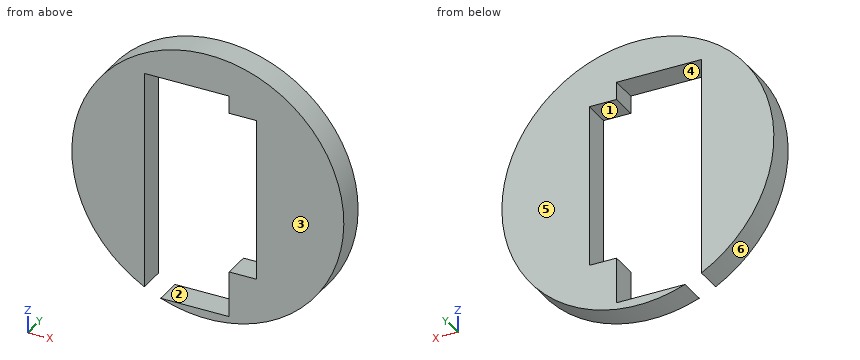
```python
from build123d import *

# Parameters (mm, degrees)
SKETCH1_R           = 47.625
BOSS_EXTRUDE1_DEPTH = 12.7
SKETCH2_R           = 47.625
BOSS_EXTRUDE4_DEPTH = 12.7
BOSS_EXTRUDE5_DEPTH = 4.7625
SKETCH14_W          = 19.812
SKETCH14_H          = 52.959
CUT_EXTRUDE11_DEPTH = 9.275815586
BOSS_EXTRUDE7_DEPTH = 6.35


with BuildPart() as part:
    # Sketch1 → Boss-Extrude1 (new body)
    with BuildSketch(Plane(origin=(0, 0, 0), x_dir=(1, 0, 0), z_dir=(0, 1, 0))):
        Circle(SKETCH1_R)
    extrude(amount=-BOSS_EXTRUDE1_DEPTH)

    # Sketch14 → Cut-Extrude11 (cut)
    with BuildSketch(Plane.XZ.offset(12.7)):
        with Locations((-4.92125, -3.302)):
            Rectangle(SKETCH14_W, SKETCH14_H)
    extrude(amount=-CUT_EXTRUDE11_DEPTH, mode=Mode.SUBTRACT)


with BuildPart() as body_2:
    # Sketch2 → Boss-Extrude4 (new body)
    with BuildSketch(Plane(origin=(0, 0, 0), x_dir=(1, 0, 0), z_dir=(0, 1, 0))):
        Circle(SKETCH2_R)
        with BuildLine():
            Line((30.48, 5.08), (26.035, 5.08))
            Line((26.035, 5.08), (26.035, -36.027507199))
            ThreePointArc((26.035, -36.027507199), (0, -44.45), (-26.035, -36.027507199))
            Line((-26.035, -36.027507199), (-26.035, 5.08))
            Line((-26.035, 5.08), (-30.48, 5.08))
            Line((-30.48, 5.08), (-30.48, -32.353857575))
            ThreePointArc((-30.48, -32.353857575), (-43.961440483, 6.572233308), (-19.685, 39.853522743))
            Line((-19.685, 39.853522743), (-19.685, 25.0825))
            Line((-19.685, 25.0825), (-15.24, 25.0825))
            Line((-15.24, 25.0825), (-15.24, 41.755776846))
            ThreePointArc((-15.24, 41.755776846), (0, 44.45), (15.24, 41.755776846))
            Line((15.24, 41.755776846), (15.24, 25.0825))
            Line((15.24, 25.0825), (19.685, 25.0825))
            Line((19.685, 25.0825), (19.685, 39.853522743))
            ThreePointArc((19.685, 39.853522743), (43.961440483, 6.572233308), (30.48, -32.353857575))
            Line((30.48, -32.353857575), (30.48, 5.08))
        make_face(mode=Mode.SUBTRACT)
    extrude(amount=BOSS_EXTRUDE4_DEPTH)


with BuildPart() as body_3:
    # Sketch10 → Boss-Extrude5 (new body)
    with BuildSketch(Plane(origin=(0, 0, 0), x_dir=(1, 0, 0), z_dir=(0, 1, 0))):
        with BuildLine():
            ThreePointArc((4.7625, -44.19412963), (7.475442585, -43.816894666), (10.16, -43.273281595))
            Line((10.16, -43.273281595), (10.16, 43.273281595))
            ThreePointArc((10.16, 43.273281595), (7.475442585, 43.816894666), (4.7625, 44.19412963))
            Line((4.7625, 44.19412963), (4.7625, -44.19412963))
        make_face()
    extrude(amount=BOSS_EXTRUDE5_DEPTH)


with BuildPart() as body_4:
    # Sketch18 → Boss-Extrude7 (new body)
    with BuildSketch(Plane.XZ.offset(12.7)):
        with BuildLine():
            Line((-14.82725, 23.1775), (4.98475, 23.1775))
            Line((4.98475, 23.1775), (4.98475, 19.05))
            Line((4.98475, 19.05), (11.33475, 19.05))
            Line((11.33475, 19.05), (11.33475, -19.05))
            Line((11.33475, -19.05), (4.98475, -19.05))
            Line((4.98475, -19.05), (4.98475, -29.7815))
            Line((4.98475, -29.7815), (-11.005669346, -29.7815))
            ThreePointArc((-11.005669346, -29.7815), (12.944605873, 28.991372489), (-14.82725, -28.075169767))
            Line((-14.82725, -28.075169767), (-14.82725, 23.1775))
        make_face()
    extrude(amount=BOSS_EXTRUDE7_DEPTH)


solid = body_4.part
```
Part model, mm, in its own coordinate system. Face numbers are marked on the shaded views. A direction names the side the tool comes from. Coordinates: 2 decimals unless noted, no trailing zeros. Order: outer loops, then holes, each group sorted by start corner. A loop starts at its lowest first (then second) coordinate and runs counter-clockwise, first axis right, second up. Notation, with made-up numbers: (-13.75, 73.5) - (29.25, 73.5) arc R19 cw to (29.25, 97.5) - close; hole circle Ø10 at (-25, 63.5). An arc over 180 degrees is marked (long way). Return JSON: item names as keys, results as strings. Group by question number.
Item 1: Pull direction Z, two halves, no side cores. Call the marked faces 4, 5 and 6: pulls with the +Z half, pulls with the -Z half, needs draft (parallel to the pull), parting line crosses it, or undercut.
Item 2: Cut at C-C (x = 0). List the corners of the cut face in (y, z), plus the area to 3 significant figures.
Item 3: Cut at A-A (z = -5.5). List the corners of the cut face in (x, y), plus the area to 3 significant figures.
Item 4: Which spindle directions (+Z, -Z, +X, -X, +Y, -Y) get a long thin tool onto all of the face, cutting with end or side? Do the marked faces 1, 2 and 3. Say none if no direction does.
Item 5: Cut at D-D (x = 20). List the corners of the cut face in (y, z).
Item 6: Drill centre lines: probe 1 along Z at (x, y) = (-4.5, -18.5); probe 2 along X at (y, z) = (-16.25, -4.5); probe 3 along X at (y, z) = (-15.25, 1). Where is each one in solid material? Low to high. Write a range as from..to.
Item 7: Cut at B-B (y = -13.75). List the corners of the cut face in (x, z), plus the area to 3 significant figures.
Item 8: Pin check, flat tips, straight feed: pin 1 (1.9 mm diameter, centred on y = -16, z = -23, fed in from -X); pin 2 (3.5 mm diameter, centred on y = -17, z = 21, fed in from -X); pin 3 (1.5 mm diameter, centred on x = 6.5, y = -16.5, fed in from +Z) (3 decimals). Stop position of each tip, or through.
Check values:
{
 "1": {"face 4": "undercut", "face 5": "needs draft", "face 6": "parting line crosses it"},
 "2": {"outline": "(-19.05, -31.75) - (-12.7, -31.75) - (-12.7, -29.78) - (-19.05, -29.78) - close; (-19.05, 23.18) - (-12.7, 23.18) - (-12.7, 31.75) - (-19.05, 31.75) - close", "area": "66.9 mm2"},
 "3": {"outline": "(-31.27, -19.05) - (-14.83, -19.05) - (-14.83, -12.7) - (-31.27, -12.7) - close; (11.33, -19.05) - (31.27, -19.05) - (31.27, -12.7) - (11.33, -12.7) - close", "area": "231 mm2"},
 "4": {"face 1": "+Y, -Y", "face 2": "-X, +Y, -Y", "face 3": "+Z, -Z, +X, -X, -Y"},
 "5": {"outline": "(-19.05, -24.66) - (-12.7, -24.66) - (-12.7, 24.66) - (-19.05, 24.66) - close"},
 "6": {"probe 1": "z = -31.43..-29.78, 23.18..31.43", "probe 2": "x = -31.43..-14.83, 11.33..31.43", "probe 3": "x = -31.73..-14.83, 11.33..31.73"},
 "7": {"outline": "(-14.83, -28.08) - (-14.83, 23.18) - (4.98, 23.18) - (4.98, 19.05) - (11.33, 19.05) - (11.33, -19.05) - (4.98, -19.05) - (4.98, -29.78) - (-11.01, -29.78) arc R31.75 ccw (long way) to start", "area": "1,880 mm2"},
 "8": {"pin 1": "stops at x = -22.84", "pin 2": "stops at x = -25.25", "pin 3": "stops at z = 31.225"}
}
